Here's how the part is built. I have some questions about the finished solid (model axes, mm). A direction names the side the tool comes from. Round coordinates to 2 decimals unless told otherwise and drop trailing zeros. Order: outer loops, then holes, each group sorted by start corner. A loop starts at its lowest first (then second) coordinate and runs counter-clockwise, first axis right, second up.
```python
from build123d import *

# Parameters (mm, degrees)
F0_W     = 285
F0_H     = 195
F1_DEPTH = 100
F2_T     = -1
F3_D     = 4.1


# Not quite as in the source:
# - a feature names something its author has since deleted; it is built from what else it names


with BuildPart() as f1:
    # F0 (on Top) → F1 (new body)
    with BuildSketch(Plane.XY):
        with Locations((12.5, 2.5)):
            Rectangle(F0_W, F0_H)
    extrude(amount=F1_DEPTH)

    # F2
    f2_openings = [f1.faces().sort_by_distance(p)[0] for p in [
        (12.5, 2.5, 100),
    ]]
    offset(amount=F2_T, openings=f2_openings)

    # F3 (through all)
    with Locations(Plane(origin=(0, 0, 0), x_dir=(1, 0, 0), z_dir=(0, 0, -1))):
        with Locations((15, -88), (-118, -88), (143, 83), (-118, 83)):
            Hole(F3_D / 2)


solid = f1.part
```
1. I need wall thicknesses on probe 1 along X at (y, z) = (-83, 0.55); probe 2 along Y at (x, z) = (-118, 0.3); probe 3 along Y at (x, z) = (-69, 45.5). Which ranges of each line are inside material? Lowest first, please.
Evaluation:
probe 1: x = -130 to -120.05, -115.95 to 140.95, 145.05 to 155
probe 2: y = -95 to -85.05, -80.95 to 85.95, 90.05 to 100
probe 3: y = -95 to -94, 99 to 100
2. If we mould it in two halves opening along X, with no side actions, what happens to faces 1 (the flat face through (11, 4, 0)), 2 (the flat face through (-130, 1, 49)), 3 (the flat face through (-129, 1, 50))? For each: released by +X, released by -X, zero draft, split by the parting line, or undercut.
Evaluation:
face 1: zero draft
face 2: released by -X
face 3: undercut
3. If we section it at C-C, the plane x = 99.5: Write out the boundary of the cut face in (y, z).
Evaluation:
outline: (-95, 0) - (100, 0) - (100, 100) - (99, 100) - (99, 1) - (-94, 1) - (-94, 100) - (-95, 100) - close
4. I'm going to push a flat-ended pin straight in: P1, Ø5, axis at x = -73.5, y = -18.5, coming from the +Z side. Where does the tip first touch, or does it pass through?
Evaluation:
P1: stops at z = 1
5. On a 3-axis mill with a long thin cutter (end or side, diameter ignored), from which of +Z, -Z, +X, -X, +Y, -Y can I reach the whole of each face in a straight line? I mean faces 4 (the flat face through (11, -95, 49)), 5 (the flat face through (11, 4, 1)). Say none if no direction works.
Evaluation:
face 4: +Z, -Z, +X, -X, -Y
face 5: +Z
6. If we section it at A-A, the plane z = 33: Write out the boundary of the cut face in (x, y).
Evaluation:
outline: (-130, -95) - (155, -95) - (155, 100) - (-130, 100) - close; hole (-129, -94) - (154, -94) - (154, 99) - (-129, 99) - close
7. If we section it at B-B, the plane y = -14.5: Write out the boundary of the cut face in (x, z), and give its area (3 significant figures).
Evaluation:
outline: (-130, 0) - (155, 0) - (155, 100) - (154, 100) - (154, 1) - (-129, 1) - (-129, 100) - (-130, 100) - close
area: 483 mm2
